The listing builds one solid part. Answer for the finished solid, in the listing's coordinates (mm). A direction names the side the tool comes from. Coordinates: 2 decimals unless noted, no trailing zeros. Write each loop counter-clockwise with the first axis right and the second up, starting at its lowest first coordinate (ties: lowest second). Pieces come first, ordered by that corner, then holes.
Autodesk Inventor part; units mm, degrees
ref_plane "Work Plane1" through (0, 0, 72.3) normal (0, 0, 1) x (1, 0, 0)
ref_plane "YZ Plane" through (0, 0, 0) normal (1, 0, 0) x (0, 1, 0)
ref_plane "XZ Plane" through (0, 0, 0) normal (0, 1, 0) x (-1, 0, 0)
sketch "Sketch1" plane through (0, 0, 0) normal (0, 0, 1) x (1, 0, 0)
  circle A0 centre (0, 0) radius 12.5
  dimension "d0" = 25
extrude "Extrusion1" add sketch "Sketch1" along normal blind 5.3
sketch "Sketch2" plane through (0, 0, 5.3) normal (0, 0, 1) x (1, 0, 0)
  circle A0 centre (0, 0) radius 18
  dimension "d3" = 36
extrude "Extrusion2" add sketch "Sketch2" along normal blind 29.8
sketch "Sketch3" plane through (0, 0, 35.1) normal (0, 0, 1) x (1, 0, 0)
  circle A0 centre (0, 0) radius 19.5
  dimension "d6" = 39
extrude "Extrusion3" add sketch "Sketch3" along normal blind 8
sketch "Sketch4" plane through (0, 0, 43.1) normal (0, 0, 1) x (1, 0, 0)
  circle A0 centre (0, 0) radius 18.2
  dimension "d9" = 36.4
extrude "Extrusion4" add sketch "Sketch4" along normal blind 17.2
sketch "Sketch5" plane through (0, 0, 60.3) normal (0, 0, 1) x (1, 0, 0)
  circle A0 centre (0, 0) radius 16.45
  dimension "d12" = 32.9
extrude "Extrusion5" add sketch "Sketch5" along normal blind 1.8
sketch "Sketch6" plane through (0, 0, 62.1) normal (0, 0, 1) x (1, 0, 0)
  circle A0 centre (0, 0) radius 16.45
  dimension "d15" = 32.9
extrude "Extrusion6" add sketch "Sketch6" along normal blind 6.8
sketch "Sketch7" plane through (0, 0, 68.9) normal (0, 0, 1) x (1, 0, 0)
  circle A0 centre (0, 0) radius 16.45
  dimension "d18" = 32.9
ref_plane "Work Plane1" through (0, 0, 72.3) normal (0, 0, 1) x (1, 0, 0)
sketch "Sketch8" plane through (0, 0, 72.3) normal (0, 0, 1) x (1, 0, 0)
  circle A0 centre (0, 0) radius 10.75
  dimension "d20" = 21.5
loft "Loft1" add profiles "Sketch8" section 1 edges at (-16.45, 0, 68.9)
sketch "Sketch9" plane through (0, 0, 72.3) normal (0, 0, 1) x (1, 0, 0)
  circle A0 centre (0, 0) radius 8.45
  dimension "d25" = 16.9
extrude "Extrusion7" cut sketch "Sketch9" against normal blind 1
properties part number "olympusXLSLPLN25XGMP_vFIN"
1. Find the intervals of material crossed by L1, parallel to Z at x = 0, y = 0; L2, parallel to Y at x = 0, z = 71.95; L3, parallel to Z at x = -2, y = 16.5, in increasing order.
Results found:
L1: z = 0 to 71.3
L2: y = -11.34 to -8.45, 8.45 to 11.34
L3: z = 5.3 to 60.3
2. Section C-C on z = 37 is taken. Give the vertices of the cut face in (x, y), then the cut area to 3 significant figures.
Results found:
outline: circle Ø39 at (0, 0)
area: 1,190 mm2
3. For a pull along Y with two mould halves and no side action, classify faces 4 (the cylindrical face through (-3.566, 16.059, 64.54)), 5 (the flat face through (-14, -9, 60.3)), 6 (the cylindrical face through (8.06, 2.54, 71.81)) as pulls with the +Y half, pulls with the -Y half, needs draft (parallel to the pull), parting line crosses it, or undercut.
Results found:
face 4: parting line crosses it
face 5: needs draft
face 6: undercut
4. Flat-ended cylindrical pins translate along their axes: P1, Ø2, axis at x = 13.5, y = 6, coming from the -Z side; P2, Ø6, axis at y = 2, z = 54, coming from the +X side; P3, Ø10, axis at x = 9.5, z = 61, coming from the +Y side. Find the tip coordinate at first contact, or state that the pin passes through.
Results found:
P1: stops at z = 5.3
P2: stops at x = 18.2
P3: stops at y = 17.62
5. Section B-B on z = 8 is taken. Give the vertices of the cut face in (x, y), then the cut area to 3 significant figures.
Results found:
outline: circle Ø36 at (0, 0)
area: 1,020 mm2
6. Section A-A on x = 0 is taken. Give the vertices of the cut face in (y, z).
Results found:
outline: (-19.5, 35.1) - (-18, 35.1) - (-18, 5.3) - (-12.5, 5.3) - (-12.5, 0) - (12.5, 0) - (12.5, 5.3) - (18, 5.3) - (18, 35.1) - (19.5, 35.1) - (19.5, 43.1) - (18.2, 43.1) - (18.2, 60.3) - (16.45, 60.3) - (16.45, 68.9) - (10.75, 72.3) - (8.45, 72.3) - (8.45, 71.3) - (-8.45, 71.3) - (-8.45, 72.3) - (-10.75, 72.3) - (-16.45, 68.9) - (-16.45, 60.3) - (-18.2, 60.3) - (-18.2, 43.1) - (-19.5, 43.1) - close
7. A tool of negligible diameter and unlimited length cuts with its end or side. For faces 1 (the flat face through (0, 0, 0)), 2 (the cylindrical face through (-2.343, -17.847, 19.991)), 3 (the flat face through (0, 0, 71.3)), from which of +Z, -Z, +X, -X, +Y, -Y can it reach the whole face along a straight path? Write none if from no direction.
Results found:
face 1: -Z, +X, -X, +Y, -Y
face 2: -Z
face 3: +Z
